from build123d import *

# Parameters (mm, degrees)
BOSS_EXTRUDE1_DEPTH = 9.525


with BuildPart() as part:
    # Sketch1 → Boss-Extrude1 (new body)
    with BuildSketch(Plane.XZ.offset(-384.4690372)):
        with BuildLine():
            Line((1658.231590128, -268.886195663), (2113.481590128, -268.886195663))
            Line((2113.481590128, -268.886195663), (2113.481590128, -237.936195663))
            ThreePointArc((2113.481590128, -237.936195663), (1900.365161789, 276.572375998), (1385.856590128, 489.688804337))
            Line((1385.856590128, 489.688804337), (845.381590128, 489.688804337))
            Line((845.381590128, 489.688804337), (845.381590128, 34.438804337))
            Line((845.381590128, 34.438804337), (1385.856590128, 34.438804337))
            ThreePointArc((1385.856590128, 34.438804337), (1578.454799653, -45.337986138), (1658.231590128, -237.936195663))
            Line((1658.231590128, -237.936195663), (1658.231590128, -268.886195663))
        make_face()
        with BuildLine():
            Line((1782.731590128, -237.936195663), (1784.731590128, -237.936195663))
            ThreePointArc((1784.731590128, -237.936195663), (1787.293243272, -238.995861932), (1786.228780262, -236.436198295))
            ThreePointArc((1786.228780262, -236.436198295), (1668.964467645, 45.171681854), (1387.356587496, 162.435994471))
            ThreePointArc((1387.356587496, 162.435994471), (1384.796923859, 163.500457481), (1385.856590128, 160.938804337))
            Line((1385.856590128, 160.938804337), (1385.856590128, 158.938804337))
            ThreePointArc((1385.856590128, 158.938804337), (1384.794924432, 156.379150643), (1387.356587429, 157.435958937))
            ThreePointArc((1387.356587429, 157.435958937), (1665.428933739, 41.636147948), (1781.228744728, -236.436198362))
            ThreePointArc((1781.228744728, -236.436198362), (1780.171936434, -238.997861359), (1782.731590128, -237.936195663))
        make_face(mode=Mode.SUBTRACT)
        with BuildLine():
            Line((1993.481590128, -237.936195663), (1995.481590128, -237.936195663))
            ThreePointArc((1995.481590128, -237.936195663), (1998.042900945, -238.99620479), (1996.979749261, -236.436196793))
            ThreePointArc((1996.979749261, -236.436196793), (1817.98722178, 194.194435989), (1387.356588998, 373.186963469))
            ThreePointArc((1387.356588998, 373.186963469), (1384.796581001, 374.250115154), (1385.856590128, 371.688804337))
            Line((1385.856590128, 371.688804337), (1385.856590128, 369.688804337))
            ThreePointArc((1385.856590128, 369.688804337), (1384.795273945, 367.128800582), (1387.356588979, 368.186948284))
            ThreePointArc((1387.356588979, 368.186948284), (1814.451687874, 190.658902083), (1991.979734075, -236.436196812))
            ThreePointArc((1991.979734075, -236.436196812), (1990.921586373, -238.997511846), (1993.481590128, -237.936195663))
        make_face(mode=Mode.SUBTRACT)
        with BuildLine():
            Line((1923.231590128, -237.936195663), (1925.231590128, -237.936195663))
            ThreePointArc((1925.231590128, -237.936195663), (1927.792985423, -238.996120202), (1926.729510165, -236.436197105))
            ThreePointArc((1926.729510165, -236.436197105), (1768.312970402, 144.520184611), (1387.356588686, 302.936724374))
            ThreePointArc((1387.356588686, 302.936724374), (1384.796665589, 304.000199632), (1385.856590128, 301.438804337))
            Line((1385.856590128, 301.438804337), (1385.856590128, 299.438804337))
            ThreePointArc((1385.856590128, 299.438804337), (1384.795187976, 296.878886664), (1387.356588659, 297.936704967))
            ThreePointArc((1387.356588659, 297.936704967), (1764.777436496, 140.984650705), (1921.729490758, -236.436197132))
            ThreePointArc((1921.729490758, -236.436197132), (1920.671672455, -238.997597815), (1923.231590128, -237.936195663))
        make_face(mode=Mode.SUBTRACT)
        with BuildLine():
            Line((1852.981590128, -237.936195663), (1854.981590128, -237.936195663))
            ThreePointArc((1854.981590128, -237.936195663), (1857.543095111, -238.996010351), (1856.47919969, -236.436197568))
            ThreePointArc((1856.47919969, -236.436197568), (1718.638719024, 94.845933233), (1387.356588223, 232.686413898))
            ThreePointArc((1387.356588223, 232.686413898), (1384.796775441, 233.75030932), (1385.856590128, 231.188804337))
            Line((1385.856590128, 231.188804337), (1385.856590128, 229.188804337))
            ThreePointArc((1385.856590128, 229.188804337), (1384.795076077, 226.628998732), (1387.356588182, 227.686388229))
            ThreePointArc((1387.356588182, 227.686388229), (1715.103185118, 91.310399327), (1851.47917402, -236.436197609))
            ThreePointArc((1851.47917402, -236.436197609), (1850.421784523, -238.997709714), (1852.981590128, -237.936195663))
        make_face(mode=Mode.SUBTRACT)
    extrude(amount=BOSS_EXTRUDE1_DEPTH)


solid = part.part
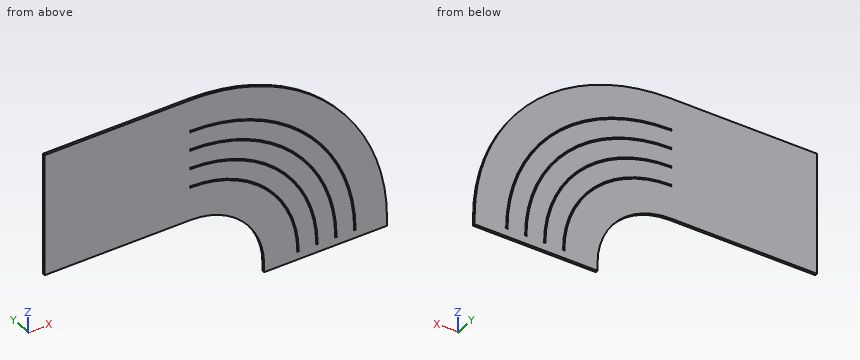
Design review of the part built by this model. Coordinates are the model's own, in mm. Round coordinates to 2 decimals unless told otherwise and drop trailing zeros. Write each loop counter-clockwise with the first axis right and the second up, starting at its lowest first coordinate (ties: lowest second). Pieces come first, ordered by that corner, then holes. Notation, with made-up numbers: M 13.25,33 L 45.25,33 A29 ccw 45.25,71 Z; hole C -10,18.5 d1. An arc over 180 degrees is marked long. One line per item, written item: value. Start each with the question number.
1. Take a section at A-A on x = 1712. State the section outline as (y, z) points, then the cut area to 3 significant figures.
2. Take a section at C-C on z = 19. State the section outline as (x, y) points, then the cut area to 3 significant figures.
3. Take a section at B-B on z = 190. State the section outline as (x, y) points, then the cut area to 3 significant figures.
4. To check wall thickness, follow probe 1 along X at (y, z) = (382, -83.5); probe 2 along X at (y, z) = (379.25, 112); probe 3 along Z at (x, y) = (1043.5, 378.5). State the ranges of each line that lie inside material, in increasing order. Write a range as from..to.
5. Take a section at D-D on y = 378.5. State how many separate pieces and enclosed holes the cut face has, then the cut area to 3 significant figures.
6. Clearance check with flat-ended pins moving along their axes: P1, Ø0.6, axis at x = 1854, y = 379.5, coming from the +Z side; P2, Ø1.6, axis at y = 377.5, z = 370.5, coming from the +X side; P3, Ø1, axis at x = 1784, y = 379.5, coming from the +Z side; P4, Ø5, axis at x = 1494, z = 363, coming from the -Y side. State where each tip first meets the part, or that it passes through.
Computed:
1. outline: M 374.94,-268.89 L 384.47,-268.89 L 384.47,-14.44 L 374.94,-14.44 Z; M 374.94,-5.71 L 384.47,-5.71 L 384.47,94.38 L 374.94,94.38 Z; M 374.94,101.35 L 384.47,101.35 L 384.47,187.26 L 374.94,187.26 Z; M 374.94,193.55 L 384.47,193.55 L 384.47,272.96 L 374.94,272.96 Z; M 374.94,278.89 L 384.47,278.89 L 384.47,412.5 L 374.94,412.5 Z
1. area: 6,220 mm²
2. outline: M 1476.26,374.94 L 1686.36,374.94 L 1686.36,384.47 L 1476.26,384.47 Z; M 1692.91,374.94 L 1774.17,374.94 L 1774.17,384.47 L 1692.91,384.47 Z; M 1780.16,374.94 L 1856.12,374.94 L 1856.12,384.47 L 1780.16,384.47 Z; M 1861.81,374.94 L 1934.83,374.94 L 1934.83,384.47 L 1861.81,384.47 Z; M 1940.35,374.94 L 2066.61,374.94 L 2066.61,384.47 L 1940.35,384.47 Z
2. area: 5,400 mm²
3. outline: M 845.38,374.94 L 1569.37,374.94 L 1569.37,384.47 L 845.38,384.47 Z; M 1581.71,374.94 L 1708.4,374.94 L 1708.4,384.47 L 1581.71,384.47 Z; M 1716.64,374.94 L 1815.11,374.94 L 1815.11,384.47 L 1716.64,384.47 Z; M 1822.14,374.94 L 1974.34,374.94 L 1974.34,384.47 L 1822.14,384.47 Z
3. area: 10,500 mm²
4. probe 1: x = 1610.22..1749.82, 1755.25..1825.12, 1830.42..1899, 1904.21..1971.98, 1977.15..2096.9
4. probe 2: x = 845.38..1569.88, 1580.39..1693.02, 1700.55..1791.7, 1798.28..1880.76, 1886.87..2023.81
4. probe 3: z = 34.44..489.69
5. separate pieces: 1
5. enclosed holes: 4
5. area: 602,000 mm²
6. P1: stops at z = 319.34
6. P2: stops at x = 1786.13
6. P3: stops at z = 371.42
6. P4: stops at y = 374.94
